Here's the drawing with two shaded views (mm, measured from the low corner). I have some questions. A direction names the side the tool comes from. Give positions to 0.01 mm unless a question says otherwise; leave off trailing zeros. Loops run counter-clockwise (first coordinate to the right, second up) from the corner with the lowest first, then second, coordinate; pieces in that order, holes last. Notation, with made-up numbers: M 61.5,-36 L 71.5,-36 A20 ccw 71.5,-4 Z; hole C -7,23.5 d7. An arc over 180 degrees is marked long. Answer in a Markdown table with one row per item. Add a question column.
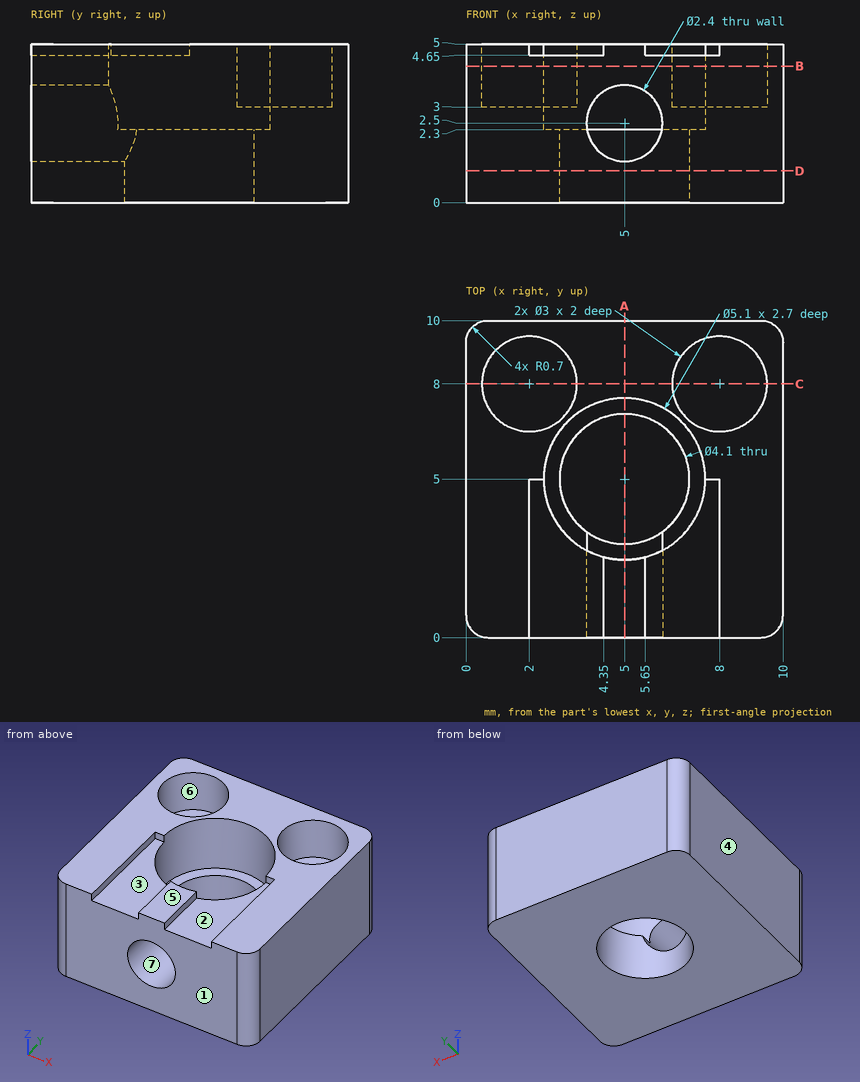
Item 1: Suppose I cut it at C-C (y = 8). List the corners of the cut face in (x, z) for me.
Item 2: I need wall thicknesses on L1, parallel to Y at x = 5, z = 0.95; L2, parallel to Y at x = 8, z = 3.45; L3, parallel to Z at x = 5, y = 1.95. Which ranges of each line are inside material? Lowest first, please.
Item 3: Suppose I cut it at D-D (z = 1). List the corners of the cut face in (x, y) for me.
Item 4: For the marked faces 5, 6 and 7, which set-ups out of +Z, -Z, +X, -X, +Y, -Y let a thin tool reach every point of the face, with its end or its side?
Item 5: Suppose I cut it at A-A (x = 5). List the corners of the cut face in (y, z) for me, then the cut area to 3 significant figures.
Item 6: Suppose I cut it at B-B (z = 4.3). List the corners of the cut face in (x, y) for me, then the cut area to 3 significant figures.
Item 7: If we mould it in two halves opening along X, with no side actions, what happens to the marked faces 1, 2, 3 and 4? For each: +X half, -X half, draft (parallel to the pull), parting line (faces both ways), or undercut.
Item 8: For P1, Ø0.9, axis at x = 8, y = 8, coming from the +Z side; P2, Ø2.5, axis at x = 3, y = 3.5, coming from the +Z side; P3, Ø3.5, axis at x = 5, y = 5, coming from the -Z side; P4, Ø2.5, axis at x = 6.5, y = 3.5, coming from the +Z side, each with a flat end and sliding along its axis, tell me the tip position at first contact or that it passes through.
Values found:
| question | item | result |
|---|---|---|
| 1 | outline | M 0,0 L 10,0 L 10,5 L 9.5,5 L 9.5,3 L 6.5,3 L 6.5,5 L 3.5,5 L 3.5,3 L 0.5,3 L 0.5,5 L 0,5 Z |
| 2 | L1 | 0 to 2.95, 7.05 to 10 |
| 2 | L2 | 0 to 6.5, 9.5 to 10 |
| 2 | L3 | 0 to 1.3, 3.7 to 5 |
| 3 | outline | M 0,0.7 A0.7 ccw 0.7,0 L 9.3,0 A0.7 ccw 10,0.7 L 10,9.3 A0.7 ccw 9.3,10 L 0.7,10 A0.7 ccw 0,9.3 Z; hole C 5,5 d4.1 |
| 4 | face 5 | +Z, +X, -X, +Y, -Y |
| 4 | face 6 | +Z |
| 4 | face 7 | -Y |
| 5 | outline | M 0,0 L 2.95,0 L 2.95,1.3 L 0,1.3 Z; M 0,3.7 L 2.45,3.7 L 2.45,5 L 0,5 Z; M 7.05,0 L 10,0 L 10,5 L 7.55,5 L 7.55,2.3 L 7.05,2.3 Z |
| 5 | area | 20.4 mm² |
| 6 | outline | M 0,0.7 A0.7 ccw 0.7,0 L 9.3,0 A0.7 ccw 10,0.7 L 10,9.3 A0.7 ccw 9.3,10 L 0.7,10 A0.7 ccw 0,9.3 Z; hole C 2,8 d3; hole C 5,5 d5.1; hole C 8,8 d3 |
| 6 | area | 65.0 mm² |
| 7 | face 1 | draft |
| 7 | face 2 | undercut |
| 7 | face 3 | undercut |
| 7 | face 4 | -X half |
| 8 | P1 | z = 3 |
| 8 | P2 | z = 5 |
| 8 | P3 | through |
| 8 | P4 | z = 4.65 |
